Check sheet for the modelled part. Datum: model origin and axes. Units: mm. A direction names the side the tool comes from. Round coordinates to 2 decimals unless told otherwise and drop trailing zeros. Write each loop counter-clockwise with the first axis right and the second up, starting at its lowest first coordinate (ties: lowest second). Pieces come first, ordered by that corner, then holes. Notation, with made-up numbers: (43.25, -19) -> (54.25, -19) arc R20 cw to (54.25, -9) -> close; hole circle Ø1 at (53.5, -9.5). An arc over 180 degrees is marked (long way). One line per item, written item: value.
from build123d import *

# Parameters (mm, degrees)
SKETCH1_R               = 20
BOSS_EXTRUDE1_DEPTH     = 25
SKETCH4_R               = 20
SKETCH4_R_2             = 17
CUT_EXTRUDE1_DEPTH      = 8
CUT_EXTRUDE2_REACH      = 39.749
CUT_EXTRUDE2_END_RADIUS = 17
SKETCH5_R               = 1.5
CIRPATTERN1_COUNT       = 3


with BuildPart() as part:
    # Sketch1 → Boss-Extrude1 (new, symmetric)
    with BuildSketch(Plane.XY):
        Circle(SKETCH1_R)
    extrude(amount=BOSS_EXTRUDE1_DEPTH, both=True)

    # Sketch3 → Hole1 (revolve, cut)
    with BuildSketch(Plane(origin=(0, 0, 25), x_dir=(0, -1, 0), z_dir=(1, 0, 0))):
        Polygon((0, 0), (0, 56.609466809), (11, 50), (11, 9), (14, 9), (14, 0), align=None)
    hole1 = revolve(axis=Axis((0, 0, 36.310875039), (0, 0, -1)), mode=Mode.SUBTRACT)

    # Sketch4 → Cut-Extrude1 (cut)
    with BuildSketch(Plane.XY.offset(25)):
        Circle(SKETCH4_R)
        Circle(SKETCH4_R_2, mode=Mode.SUBTRACT)
    cut_extrude1 = extrude(amount=-CUT_EXTRUDE1_DEPTH, mode=Mode.SUBTRACT)

    # Mirror2: Hole1, Cut-Extrude1 across plane
    add(hole1.mirror(Plane.XY), mode=Mode.SUBTRACT)
    add(cut_extrude1.mirror(Plane.XY), mode=Mode.SUBTRACT)

    # Cut-Extrude2: up to this cylinder (the profile starts inside it)
    cut_extrude2_end = Plane(origin=(0, 0, 0), z_dir=(0, 0, 1)) * Cylinder(CUT_EXTRUDE2_END_RADIUS, 156.498, mode=Mode.PRIVATE)
    # Sketch5 → Cut-Extrude2 (cut, up to the surface)
    with BuildSketch(Plane(origin=(0, 0, 0), x_dir=(0, 0, -1), z_dir=(1, 0, 0)), mode=Mode.PRIVATE) as cut_extrude2_sk1:
        with Locations(Location((-21, 0, 0), (0, 0, 180))):
            Circle(SKETCH5_R)
    cut_extrude2_tool1 = extrude(cut_extrude2_sk1.sketch, amount=CUT_EXTRUDE2_REACH, mode=Mode.PRIVATE) & cut_extrude2_end
    # Sketch5 → Cut-Extrude2 (cut, up to the surface)
    with BuildSketch(Plane(origin=(0, 0, 0), x_dir=(0, 0, -1), z_dir=(1, 0, 0)), mode=Mode.PRIVATE) as cut_extrude2_sk2:
        with Locations(Location((21, 0, 0), (0, 0, 180))):
            Circle(SKETCH5_R)
    cut_extrude2_tool2 = extrude(cut_extrude2_sk2.sketch, amount=CUT_EXTRUDE2_REACH, mode=Mode.PRIVATE) & cut_extrude2_end
    cut_extrude2 = cut_extrude2_tool1.solids().sort_by_distance((0, 0, 21))[0] + cut_extrude2_tool2.solids().sort_by_distance((0, 0, -21))[0]
    add(cut_extrude2, mode=Mode.SUBTRACT)

    # CirPattern1: Cut-Extrude2 ×3 about axis
    cirpattern1_axis = Axis((0, 0, 25), (0, 0, 1))
    for i in range(1, CIRPATTERN1_COUNT):
        add(cut_extrude2.rotate(cirpattern1_axis, i * 360 / CIRPATTERN1_COUNT), mode=Mode.SUBTRACT)


solid = part.part
Item 1: Tool access check on faces 4 (the cylindrical face through (5.362, -12.932, -20.563)), 5 (the cylindrical face through (15.44, -0.07, 19.5)), 6 (the flat face through (-9, -15, 17)). Record the directions out of +Z, -Z, +X, -X, +Y, -Y that give a thin tool (end or side, any length) a straight path to the whole face; none if there is none.
Answer:
face 4: -Z
face 5: +X
face 6: +Z
Item 2: Sectioned sample at C-C on z = 12. Enter the section's corners in (x, y), and give its area (3 significant figures).
Answer:
outline: circle Ø40 at (0, 0); hole circle Ø22 at (0, 0)
area: 877 mm^2
Item 3: Sectioned sample at B-B on y = 0. Count the separate pieces of the cut face and the enclosed holes in it, and give its area (3 significant figures).
Answer:
separate pieces: 4
enclosed holes: 0
area: 678 mm^2
Item 4: Sectioned sample at A-A on x = 0. Enter the section's corners in (y, z), and give its area (3 significant figures).
Answer:
outline: (-20, -17) -> (-17, -17) -> (-17, -25) -> (-14, -25) -> (-14, -16) -> (-11, -16) -> (-11, 16) -> (-14, 16) -> (-14, 25) -> (-17, 25) -> (-17, 17) -> (-20, 17) -> close; (11, -16) -> (14, -16) -> (14, -25) -> (17, -25) -> (17, -17) -> (20, -17) -> (20, 17) -> (17, 17) -> (17, 25) -> (14, 25) -> (14, 16) -> (11, 16) -> close
area: 696 mm^2
Item 5: Sectioned sample at D-D on z = 21. Enter the section's corners in (x, y) (3 decimals), and give its area (3 significant figures).
Answer:
outline: (-9.766, -13.915) -> (-8.259, -11.305) arc R14 cw to (-8.259, 11.305) -> (-9.766, 13.915) arc R17 ccw to start; (-7.168, -15.415) arc R17 ccw to (16.934, -1.5) -> (13.919, -1.5) arc R14 cw to (-5.661, -12.805) -> close; (-7.168, 15.415) -> (-5.661, 12.805) arc R14 cw to (13.919, 1.5) -> (16.934, 1.5) arc R17 ccw to start
area: 265 mm^2
Item 6: Mould release check, pull along Y, two halves, no side actions. Record for faces 1 (the flat face through (-9, -15, -17)), 2 (the flat face through (9.3, 6.2, 16)), 3 (the cylindrical face through (-4.336, -19.524, 0.238)): pulls with the +Y half, pulls with the -Y half, needs draft (parallel to the pull), parting line crosses it, or undercut.
Answer:
face 1: needs draft
face 2: undercut
face 3: parting line crosses it
Item 7: Thickness scan on line 1 (Z direction, x = 15, y = 0); line 2 (Y direction, x = 0, z = -2.5); line 3 (Y direction, x = 0, z = 22.5). Record the ranges inside material, lowest first.
Answer:
line 1: z = -25 to -22.5, -19.5 to 19.5, 22.5 to 25
line 2: y = -20 to -11, 11 to 20
line 3: y = -17 to -14, 14 to 17
Item 8: Depth check by flat-ended pin: P1, Ø22.5, axis at x = 0, y = 1, coming from the +Z side; P2, Ø22.5, axis at x = 1.5, y = -2, coming from the -Z side; P3, Ø6, axis at x = 1.5, z = -14.5, coming from the +Y side. Enter the tip coordinate at first touch or a pass-through.
Answer:
P1: stops at z = 16
P2: stops at z = -16
P3: stops at y = 20
